Verification items for the finished model (mm, model axes). A direction names the side the tool comes from. Give positions to 0.01 mm unless a question says otherwise; leave off trailing zeros. Loops run counter-clockwise (first coordinate to the right, second up) from the corner with the lowest first, then second, coordinate; pieces in that order, holes last. Notation, with made-up numbers: M 12.25,-5.75 L 57.25,-5.75 A19 cw 57.25,6.25 Z; hole C -22,4 d10. An arc over 180 degrees is marked long. Put each result on its own line as item: value. Start each with the question number.
from build123d import *

# Parameters (mm, degrees)
BOSS_EXTRUDE1_DEPTH  = 6.5
SKETCH2_R            = 5.5
CUT_EXTRUDE2_DEPTH   = 5
SKETCH3_R            = 4
CUT_EXTRUDE4_DEPTH   = 1.5
M2_CLEARANCE_HOLE1_D = 2.4
M2_CLEARANCE_HOLE2_D = 2.4
SKETCH8_W            = 15
SKETCH8_H            = 13
CUT_EXTRUDE5_DEPTH   = 4


with BuildPart() as part:
    # Sketch1 → Boss-Extrude1 (new body)
    with BuildSketch(Plane(origin=(0, 24.8, 0), x_dir=(1, 0, 0), z_dir=(0, 1, 0))):
        with BuildLine():
            Line((5.5, 9), (-22, 9))
            Line((-22, 9), (-22, -9))
            Line((-22, -9), (5.5, -9))
            ThreePointArc((5.5, -9), (14.5, 0), (5.5, 9))
        make_face()
    extrude(amount=BOSS_EXTRUDE1_DEPTH)

    # Sketch2 → Cut-Extrude2 (cut)
    with BuildSketch(Plane(origin=(0, 24.8, 0), x_dir=(1, 0, 0), z_dir=(0, 1, 0))):
        with Locations(Location((5.5, 0, 0), (0, 0, 270))):
            Circle(SKETCH2_R)
    extrude(amount=CUT_EXTRUDE2_DEPTH, mode=Mode.SUBTRACT)

    # Sketch3 → Cut-Extrude4 (cut)
    with BuildSketch(Plane(origin=(0, 29.8, 0), x_dir=(1, 0, 0), z_dir=(0, 1, 0))):
        with Locations(Location((5.5, 0, 0), (0, 0, 270))):
            Circle(SKETCH3_R)
    extrude(amount=CUT_EXTRUDE4_DEPTH, mode=Mode.SUBTRACT)

    # M2 Clearance Hole1 (through all)
    with Locations(Plane(origin=(0, 31.3, 0), x_dir=(1, 0, 0), z_dir=(0, 1, 0))):
        with Locations((-19.5, -4.5)):
            Hole(M2_CLEARANCE_HOLE1_D / 2)

    # M2 Clearance Hole2 (through all)
    with Locations(Plane(origin=(0, 31.3, 0), x_dir=(1, 0, 0), z_dir=(0, 1, 0))):
        with Locations((-19.5, 4.5)):
            Hole(M2_CLEARANCE_HOLE2_D / 2)

    # Sketch8 → Cut-Extrude5 (cut)
    with BuildSketch(Plane(origin=(0, 31.3, 0), x_dir=(1, 0, 0), z_dir=(0, 1, 0))):
        with Locations((-9, 0)):
            Rectangle(SKETCH8_W, SKETCH8_H)
    extrude(amount=-CUT_EXTRUDE5_DEPTH, mode=Mode.SUBTRACT)


solid = part.part
Q1. Go/stop test with flat-tipped pins: pin 1 (10.5 mm diameter, centred on x = 5.5, z = 0, fed in from +Y); pin 2 (6.5 mm diameter, centred on x = -11, z = 1.5, fed in from +Y); pin 3 (3.5 mm diameter, centred on x = 3, z = -0.5, fed in from -Y). Record where each tip stops, or that it passes through.
Q2. Cross-section at C-C, the plane x = -19.5. Record the boundary of the cut face in (y, z).
Q3. Cross-section at B-B, the plane y = 29.25. Record the boundary of the cut face in (x, z).
Q4. Set-up check for faces 1 (the face through (-18.3, 28, -4.55)), 2 (the face through (1, 29.8, 0)), 3 (the face through (-1.5, 29, 0)): record each of +Z, -Z, +X, -X, +Y, -Y from which the full face is reachable in a straight line by a thin tool's end or side.
Q5. Release check for a two-part mould opening along X. For faces 4 (the face through (0, 31.3, 0)), 5 (the face through (1.595, 30.54, -0.867)), 6 (the face through (-22, 28, 0)) record: pulls with the +X half, pulls with the -X half, needs draft (parallel to the pull), parting line crosses it, or undercut.
Q6. Cross-section at D-D, the plane x = -2. Record the boundary of the cut face in (y, z), then the cut area to 3 significant figures.
Q7. Scan lines: L1, parallel to Z at x = -19.5, y = 30; L2, parallel to X at y = 27.5, z = 0; L3, parallel to X at y = 30.55, z = 0. Record each from-to range of solid material in increasing order.
Q8. Cross-section at A-A, the plane z = 0. Record the boundary of the cut face in (x, y).
Ans:
1. pin 1: stops at y = 31.3
1. pin 2: stops at y = 27.3
1. pin 3: stops at y = 29.8
2. outline: M 24.8,-9 L 31.3,-9 L 31.3,-5.7 L 24.8,-5.7 Z; M 24.8,-3.3 L 31.3,-3.3 L 31.3,3.3 L 24.8,3.3 Z; M 24.8,5.7 L 31.3,5.7 L 31.3,9 L 24.8,9 Z
3. outline: M -22,-9 L 5.5,-9 A9 ccw 5.5,9 L -22,9 Z; hole C -19.5,-4.5 d2.4; hole C -19.5,4.5 d2.4; hole M -16.5,-6.5 L -1.5,-6.5 L -1.5,6.5 L -16.5,6.5 Z; hole C 5.5,0 d11
4. face 1: +Y, -Y
4. face 2: -Y
4. face 3: +Y
5. face 4: needs draft
5. face 5: undercut
5. face 6: pulls with the -X half
6. outline: M 24.8,-9 L 31.3,-9 L 31.3,-6.5 L 27.3,-6.5 L 27.3,6.5 L 31.3,6.5 L 31.3,9 L 24.8,9 Z
6. area: 65.0 mm^2
7. L1: z = -9 to -5.7, -3.3 to 3.3, 5.7 to 9
7. L2: x = -22 to -16.5, -1.5 to 0, 11 to 14.5
7. L3: x = -22 to -16.5, -1.5 to 1.5, 9.5 to 14.5
8. outline: M -22,24.8 L 0,24.8 L 0,29.8 L 1.5,29.8 L 1.5,31.3 L -1.5,31.3 L -1.5,27.3 L -16.5,27.3 L -16.5,31.3 L -22,31.3 Z; M 9.5,29.8 L 11,29.8 L 11,24.8 L 14.5,24.8 L 14.5,31.3 L 9.5,31.3 Z
